Part model, mm, in its own coordinate system. A direction names the side the tool comes from. Coordinates: 2 decimals unless noted, no trailing zeros. Use a Markdown table: item, result. Add a question column.
Q1. Tool access for faces 1 (the flat face through (-9.525, -4, -5)), 2 (the flat face through (26, -4, 3.175)), 3 (the cylindrical face through (-0.067, -18.145, 4.13)): list every direction of +Z, -Z, +X, -X, +Y, -Y with a clear straight run to the whole face (end or side of a thin tool).
Q2. Slice it at A-A on y = -12.7. Count the separate pieces of the cut face and the enclosed holes in it, then the cut area to 3 significant figures.
Q3. Pin check, flat tips, straight feed: pin 1 Ø8 at (y, z) = (-8.5, 1.5) entering from -X; pin 2 Ø6 at (x, z) = (13.5, -2.5) entering from -Y; pin 3 Ø5 at (x, z) = (26.5, -5) entering from -Y; pin 4 Ø3.5 at (x, z) = (-0.5, -3) entering from -Y. Stop position of each tip, or through.
Q4. Mould opens along X. For faces 4 (the cylindrical face through (-37.15, -18.14, 4.74)), 5 (the cylindrical face through (3.86, 14.92, -3.09)), 6 (the cylindrical face through (-7.177, -14.894, -3.662)) say: released by +X, released by -X, zero draft, split by the parting line, or undercut.
Q5. Wall check: L1, parallel to Y at x = -7.5, z = -2; L2, parallel to X at y = 13, z = 3; L3, parallel to X at y = 1, z = -7.5 (1 decimal). Give the ranges that are in metal, low to high. Write a range as from..to.
from build123d import *

# Parameters (mm, degrees)
SKETCH1_W             = 19.05
SKETCH1_H             = 38.1
BOSS_EXTRUDE1_DEPTH   = 38.1
SKETCH2_W             = 9.525
SKETCH2_H             = 34.925
CUT_EXTRUDE1_DEPTH    = 12.7
SKETCH3_W             = 28.575
SKETCH3_H             = 33.3375
CUT_EXTRUDE2_DEPTH    = 12.7
FILLET1_R             = 3.175
F_8_CLEARANCE_HOLE1_D = 4.4958
FILLET2_R             = 3.175


with BuildPart() as part:
    # Sketch1 → Boss-Extrude1 (new, symmetric)
    with BuildSketch(Plane(origin=(0, 0, 0), x_dir=(0, 0, -1), z_dir=(1, 0, 0))):
        Rectangle(SKETCH1_W, SKETCH1_H)
    extrude(amount=BOSS_EXTRUDE1_DEPTH, both=True)

    # Sketch2 → Cut-Extrude1 (cut)
    with BuildSketch(Plane(origin=(0, 0, -9.525), x_dir=(-1, 0, 0), z_dir=(0, 0, -1))):
        with Locations((0, -1.5875)):
            Rectangle(SKETCH2_W, SKETCH2_H)
    extrude(amount=-CUT_EXTRUDE1_DEPTH, mode=Mode.SUBTRACT)

    # Sketch3 → Cut-Extrude2 (cut)
    with BuildSketch(Plane(origin=(0, 0, -9.525), x_dir=(-1, 0, 0), z_dir=(0, 0, -1))):
        with Locations((-23.8125, -2.38125)):
            Rectangle(SKETCH3_W, SKETCH3_H)
        with Locations((23.8125, -2.38125)):
            Rectangle(SKETCH3_W, SKETCH3_H)
    extrude(amount=-CUT_EXTRUDE2_DEPTH, mode=Mode.SUBTRACT)

    # Fillet1
    fillet1_edges = [part.edges().sort_by_distance(p)[0] for p in [
        (38.1, 0, 9.525),
        (38.1, -19.05, 6.35),
        (4.7625, 15.875, -3.175),
        (-4.7625, 15.875, -3.175),
        (9.525, 14.2875, -3.175),
        (23.8125, 14.2875, 3.175),
        (9.525, -2.38125, 3.175),
        (-9.525, 14.2875, -3.175),
        (-9.525, -2.38125, 3.175),
        (-23.8125, 14.2875, 3.175),
        (-38.1, -19.05, 6.35),
        (-38.1, 0, 9.525),
        (-38.1, 19.05, 0),
        (38.1, 19.05, 0),
        (0, -19.05, 9.525),
        (0, 19.05, 9.525),
    ]]
    fillet(fillet1_edges, radius=FILLET1_R)

    # #8 Clearance Hole1 (through all)
    with Locations(Plane(origin=(9.525, 0, 0), x_dir=(0, 0, -1), z_dir=(1, 0, 0))):
        with Locations((3.175, -12.7), (3.175, 6.35)):
            Hole(F_8_CLEARANCE_HOLE1_D / 2)

    # Fillet2
    fillet2_edges = [part.edges().sort_by_distance(p)[0] for p in [
        (0, -19.05, 3.175),
    ]]
    fillet(fillet2_edges, radius=FILLET2_R - 0.0001)  # a hair under: the kernel refuses the full size


solid = part.part
Recorded:
| question | item | result |
|---|---|---|
| 1 | face 1 | -Z, -X, -Y |
| 1 | face 2 | -Z, +X, -Y |
| 1 | face 3 | -Z, -Y |
| 2 | separate pieces | 3 |
| 2 | enclosed holes | 0 |
| 2 | area | 562 mm² |
| 3 | pin 1 | x = -38.1 |
| 3 | pin 2 | y = 13.4 |
| 3 | pin 3 | y = 14.29 |
| 3 | pin 4 | y = 15.81 |
| 4 | face 4 | released by -X |
| 4 | face 5 | undercut |
| 4 | face 6 | zero draft |
| 5 | L1 | -19.05..-14.62, -10.78..4.43, 8.27..19.05 |
| 5 | L2 | -38.1..-4.75, 4.75..38.1 |
| 5 | L3 | -9.5..-4.8, 4.8..9.5 |
